Geometry: see drawing. Coordinates: mm, zero at the bounding-box minimum. Round coordinates to 2 decimals unless told otherwise and drop trailing zeros. Order: outer loops, then holes, each group sorted by start corner. A loop starts at its lowest first (then second) coordinate and runs counter-clockwise, first axis right, second up. Notation, with made-up numbers: (-8, 37.25) -> (14, 37.25) arc R27 ccw to (14, 54.25) -> close; hole circle Ø9 at (46.5, -26). An arc over 180 degrees is marked (long way). Put each result on its own line as item: value.
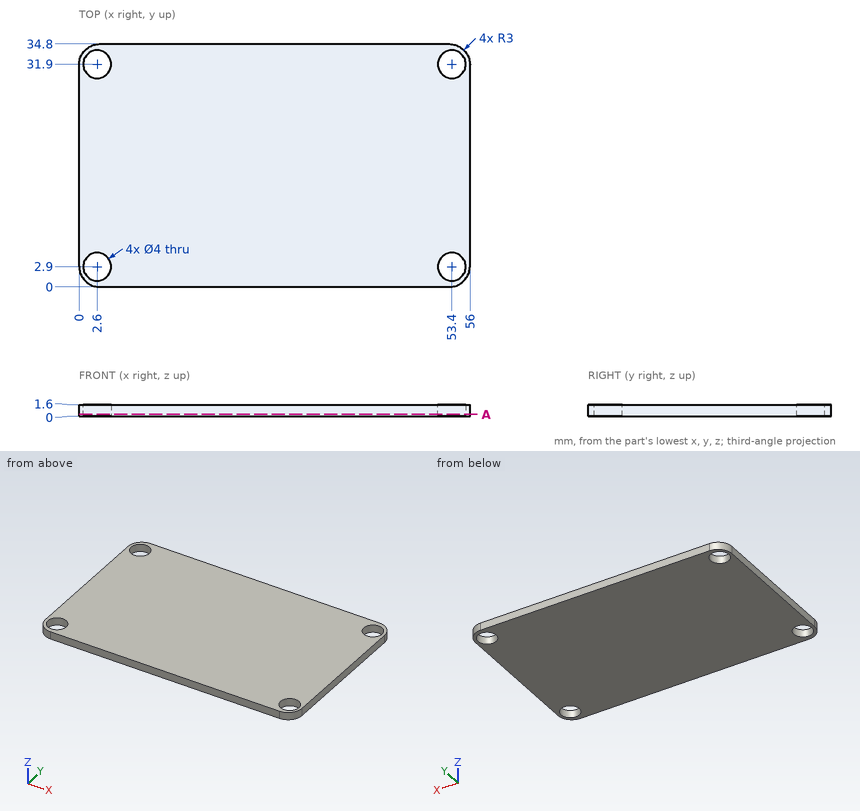
1. Material intervals for probe 1 along X at (y, z) = (3, 0.55); probe 2 along Y at (x, z) = (53.4, 0.3); probe 3 along X at (y, z) = (32.5, 1.1), sorted ascending.
Ans:
probe 1: 0 to 0.6, 4.6 to 51.4, 55.4 to 56
probe 2: 0.03 to 0.9, 4.9 to 29.9, 33.9 to 34.77
probe 3: 0.08 to 0.69, 4.51 to 51.49, 55.31 to 55.92
2. Cut plane A-A on z = 0.25. Return loops of the section in (x, y).
Ans:
outline: (0, 3) arc R3 ccw to (3, 0) -> (53, 0) arc R3 ccw to (56, 3) -> (56, 31.8) arc R3 ccw to (53, 34.8) -> (3, 34.8) arc R3 ccw to (0, 31.8) -> close; hole circle Ø4 at (2.6, 2.9); hole circle Ø4 at (2.6, 31.9); hole circle Ø4 at (53.4, 2.9); hole circle Ø4 at (53.4, 31.9)
3. Contact query for a flat-ended pin moving along its axis: P1, Ø3.5, axis at x = 53.4, y = 2.9, coming from the -Z side. Output: stop coordinate, or through.
Ans:
P1: through
